Input: part model. Units: mm. Frame: model coordinates. A direction names the side the tool comes from. Give positions to 0.01 mm unless a question says otherwise; leave off trailing zeros. Loops run counter-clockwise (first coordinate to the right, second up) from the corner with the lowest first, then second, coordinate; pieces in that order, holes last. Notation, with made-up numbers: (-35, 85) - (-9, 85) arc R19 cw to (-9, 106) - close; hole circle Ø4 at (29, 57.25). An arc over 180 degrees is marked (long way). Answer as a JSON object with one key per item and string values. Group by question number.
(1) Section query A-A (z = -6). Return loops of the section in (x, y), plus the area to 3 significant figures.
(2) Mould query, pull axis Z, two halves, no side actions, for faces 1 (the flat face through (-10, 7.5, -17)), 2 (the cylindrical face through (12.93, 11.32, -0.63)), 3 (the cylindrical face through (10, 13, -6)). Classes: +Z half, -Z half, draft (parallel to the pull), parting line (faces both ways), or undercut.
(3) Pin query (flat end, axial travel): P1, Ø1.9, axis at x = 11.5, z = -10.5, coming from the -Y side; P2, Ø4.5, axis at y = 18, z = -18.5, coming from the -X side; P3, Ø1.5, axis at x = 8.5, y = -4, coming from the -Z side; P4, Ø3, axis at y = 15, z = -6, coming from the +X side. Return the tip coordinate at first contact, or that it passes through.
(4) Section query C-C (x = -13.5). Return loops of the section in (y, z), plus the area to 3 significant figures.
(5) Section query B-B (y = 0). Return loops of the section in (x, z), plus the area to 3 significant figures.
(6) Section query D-D (z = -15). Return loops of the section in (x, y).
(7) Material intervals for L1, parallel to X at y = 0, z = 1.4; L2, parallel to Z at x = -11.1, y = 15; L3, parallel to Y at x = -9.8, z = -6, sorted ascending.
(8) Access query for faces 4 (the flat face through (-7.65, 15, -15)), 5 (the cylindrical face through (-22.124, 7.111, 2.535)). Directions: +Z, -Z, +X, -X, +Y, -Y. A direction counts if a zero-diameter tool reaches every point of the face in a straight line with its end or side. Return the directions, or none.
```python
from build123d import *

# Parameters (mm, degrees)
SKETCH1_W                         = 45
SKETCH1_H                         = 15
BOSS_EXTRUDE1_DEPTH               = 5
BOSS_EXTRUDE2_DEPTH               = 15
F_4_0_4_DIAMETER_HOLE1_AT_2_COUNT = 2
F_4_0_4_DIAMETER_HOLE1_AT_2_PITCH = 18
F_4_0_4_DIAMETER_HOLE2_AT_2_COUNT = 2
F_4_0_4_DIAMETER_HOLE2_AT_2_PITCH = 27
FILLET1_R                         = 10
FILLET2_R                         = 1.5


with BuildPart() as part:
    # Sketch1 → Boss-Extrude1 (new body)
    with BuildSketch(Plane.XY):
        Rectangle(SKETCH1_W, SKETCH1_H)
    extrude(amount=BOSS_EXTRUDE1_DEPTH)

    # Sketch3 → Boss-Extrude2 (add)
    with BuildSketch(Plane(origin=(0, 7.5, 0), x_dir=(1, 0, 0), z_dir=(0, 1, 0))):
        Polygon((-7.65, 0), (-7.65, -5), (-12.65, -5), (-12.65, 35), (-7.65, 35), align=None)
        Polygon((7.65, -5), (12.65, -5), (12.65, 35), (7.65, 35), (7.65, 0), align=None)
    extrude(amount=BOSS_EXTRUDE2_DEPTH)

    # Sketch8 → Ø4.0 (4) Diameter Hole1 (revolve, cut)
    with BuildSketch(Plane(origin=(-12.65, 15, -24), x_dir=(0, 0, 1), z_dir=(0, 1, 0))):
        Polygon((0, 0), (0, 5), (2, 5), (2, 0.603553391), (2.25, 0), align=None)
    f_4_0_4_diameter_hole1 = revolve(axis=Axis((-19, 15, -24), (1, 0, 0)), mode=Mode.SUBTRACT)

    # Ø4.0 (4) Diameter Hole1 at 2: Ø4.0 (4) Diameter Hole1 ×2
    with Locations(*[(0, 0, i * F_4_0_4_DIAMETER_HOLE1_AT_2_PITCH) for i in range(1, F_4_0_4_DIAMETER_HOLE1_AT_2_COUNT)]):
        add(f_4_0_4_diameter_hole1, mode=Mode.SUBTRACT)

    # Mirror3: Ø4.0 (4) Diameter Hole1 across plane
    add(f_4_0_4_diameter_hole1.mirror(Plane(origin=(0, 0, 0), x_dir=(0, 0, 1), z_dir=(1, 0, 0))), mode=Mode.SUBTRACT)

    # Mirror3 copy 1 sketch → Mirror3 copy 1 (revolve, cut)
    with BuildSketch(Plane(origin=(12.65, 15, -6), x_dir=(0, 0, 1), z_dir=(0, 1, 0))):
        Polygon((0, 0), (0, -5), (2, -5), (2, -0.603553391), (2.25, 0), align=None)
    revolve(axis=Axis((19, 15, -6), (1, 0, 0)), mode=Mode.SUBTRACT)

    # Sketch12 → Ø4.0 (4) Diameter Hole2 (revolve, cut)
    with BuildSketch(Plane(origin=(13.5, 0, 5), x_dir=(0, -1, 0), z_dir=(1, 0, 0))):
        Polygon((0, 0), (0, 5), (2, 5), (2, 0.603553391), (2.25, 0), align=None)
    f_4_0_4_diameter_hole2 = revolve(axis=Axis((13.5, 0, 11.35), (0, 0, -1)), mode=Mode.SUBTRACT)

    # Ø4.0 (4) Diameter Hole2 at 2: Ø4.0 (4) Diameter Hole2 ×2
    with Locations(*[(-i * F_4_0_4_DIAMETER_HOLE2_AT_2_PITCH, 0, 0) for i in range(1, F_4_0_4_DIAMETER_HOLE2_AT_2_COUNT)]):
        add(f_4_0_4_diameter_hole2, mode=Mode.SUBTRACT)

    # Fillet1
    # the kernel refuses this fillet: 10 mm, written as the material it adds along each edge
    with BuildSketch(Plane(origin=(12.65, 7.5, 5), x_dir=(1, 0, 0), z_dir=(0, 0, -1))) as fillet1_piece_1:
        with BuildLine():
            CenterArc((10, -9.998874937), FILLET1_R, 90.859468925, 89.140531075)
            Line((0, -9.998874937), (0, 0))
            Line((0, 0), (9.85, 0))
        make_face()
    extrude(amount=5)
    with BuildSketch(Plane(origin=(-12.65, 7.5, 5), x_dir=(-1, 0, 0), z_dir=(0, 0, -1))) as fillet1_piece_2:
        with BuildLine():
            CenterArc((10, 9.998874937), FILLET1_R, 180, 89.140531075)
            Line((0, 9.998874937), (0, 0))
            Line((0, 0), (9.85, 0))
        make_face()
    extrude(amount=5)

    # Fillet2
    fillet2_edges = [part.edges().sort_by_distance(p)[0] for p in [
        (-10.15, 7.5, -35),
        (-10.15, 22.5, -35),
        (-10.15, 22.5, 5),
        (10.15, 7.5, -35),
        (10.15, 22.5, 5),
        (10.15, 22.5, -35),
        (22.5, -7.5, 2.5),
        (-22.5, -7.5, 2.5),
        (-22.5, 7.5, 2.5),
        (22.5, 7.5, 2.5),
        (12.65, 12.499437468, 0),
        (-12.65, 12.499437468, 0),
    ]]
    fillet(fillet2_edges, radius=FILLET2_R)


solid = part.part
```
Recorded:
{
 "1": {"outline": "(-12.65, 7.5) - (-7.65, 7.5) - (-7.65, 13) - (-12.05, 13) - (-12.65, 12.75) - close; (-12.65, 17.25) - (-12.05, 17) - (-7.65, 17) - (-7.65, 22.5) - (-12.65, 22.5) - close; (7.65, 7.5) - (12.65, 7.5) - (12.65, 12.75) - (12.05, 13) - (7.65, 13) - close; (7.65, 17) - (12.05, 17) - (12.65, 17.25) - (12.65, 22.5) - (7.65, 22.5) - close", "area": "110 mm^2"},
 "2": {"face 1": "draft", "face 2": "-Z half", "face 3": "undercut"},
 "3": {"P1": "stops at y = 7.5", "P2": "stops at x = -12.65", "P3": "stops at z = 0", "P4": "passes through"},
 "4": {"outline": "(-7.5, 0) - (-2, 0) - (-2, 4.4) - (-2.25, 5) - (-7.5, 5) - close; (2, 0) - (7.5, 0) - (7.5, -0.15) - (13.46, -0.15) - (13.46, 5) - (2.25, 5) - (2, 4.4) - close", "area": "85.6 mm^2"},
 "5": {"outline": "(-22.5, 0) - (-15.5, 0) - (-15.5, 4.4) - (-15.75, 5) - (-22.5, 5) - close; (-11.5, 0) - (11.5, 0) - (11.5, 4.4) - (11.25, 5) - (-11.25, 5) - (-11.5, 4.4) - close; (15.5, 0) - (22.5, 0) - (22.5, 5) - (15.75, 5) - (15.5, 4.4) - close", "area": "185 mm^2"},
 "6": {"outline": "(-12.65, 7.5) - (-7.65, 7.5) - (-7.65, 22.5) - (-12.65, 22.5) - close; (7.65, 7.5) - (12.65, 7.5) - (12.65, 22.5) - (7.65, 22.5) - close"},
 "7": {"L1": "x = -22.5 to -15.5, -11.5 to 11.5, 15.5 to 22.5", "L2": "z = -35 to -26, -22 to -8, -4 to 5", "L3": "y = 7.5 to 13, 17 to 22.5"},
 "8": {"face 4": "+Z, -Z, +Y", "face 5": "+Z, -Z, -X, +Y"}
}
